The listing builds one solid part. Answer for the finished solid, in the listing's coordinates (mm). Face numbers are marked on the shaded views. A direction names the side the tool comes from. Round coordinates to 2 decimals unless told otherwise and drop trailing zeros. Order: outer loops, then holes, each group sorted by start corner. A loop starts at its lowest first (then second) coordinate and runs counter-clockwise, first axis right, second up. Notation, with made-up numbers: (35.25, 11) -> (49.25, 11) arc R25 cw to (49.25, 50) -> close; hole circle Ø11 at (-27.5, 42.5). An arc over 180 degrees is marked (long way). Return JSON: item names as keys, results as strings. Group by question number.
(1) Each of these flat-tipped pins is pushed along its axis until it touches: pin 1 (9 mm diameter, centred on x = -0.5, y = 68, fed in from +Z); pin 2 (1.5 mm diameter, centred on x = -35.5, z = 3.5, fed in from -Y); pin 3 (11.5 mm diameter, centred on x = 0, y = -70, fed in from -Z); pin 4 (5.5 mm diameter, centred on x = 49.5, y = -49.5, fed in from -Z). Where does it stop, or does it pass through?
(2) Which of the six approach directions +Z, -Z, +X, -X, +Y, -Y give full straight-line access (tool end or side, diameter ignored) to the marked faces 1 and 2?
(3) The part is cut by section D-D (x = -37.5). Determine the outline of the cut face in (y, z), plus the area to 3 significant figures.
(4) The part is cut by section C-C (y = 70). Determine the outline of the cut face in (x, z) (3 decimals).
(5) Consider line 1 (Y direction, x = 0, z = 8.2); line 2 (Y direction, x = -4, z = 7); line 3 (Z direction, x = 38, y = -21). Determine where each line is inside the solid, lowest interval first. Write a range as [from, to].
(6) The part is cut by section A-A (x = 0). Determine the outline of the cut face in (y, z) (3 decimals), plus the area to 3 significant figures.
from build123d import *

# Parameters (mm, degrees)
SKETCH1_R                               = 100
SKETCH1_R_2                             = 40
BOSS_EXTRUDE1_DEPTH                     = 15
CBORE_FOR_M8_HEX_HEAD_BOLT1_D           = 9
CBORE_FOR_M8_HEX_HEAD_BOLT1_CBORE_D     = 18.01
CBORE_FOR_M8_HEX_HEAD_BOLT1_CBORE_DEPTH = 5.68
CIRPATTERN1_COUNT                       = 8
SKETCH5_R                               = 82.5
CUT_EXTRUDE2_DEPTH                      = 5


with BuildPart() as part:
    # Sketch1 → Boss-Extrude1 (new body)
    with BuildSketch(Plane.XY):
        Circle(SKETCH1_R)
        Circle(SKETCH1_R_2, mode=Mode.SUBTRACT)
    extrude(amount=BOSS_EXTRUDE1_DEPTH)

    # CBORE for M8 Hex Head Bolt1 (through all)
    with Locations(Plane.XY.offset(15)):
        with Locations((0, 70)):
            cbore_for_m8_hex_head_bolt1 = CounterBoreHole(CBORE_FOR_M8_HEX_HEAD_BOLT1_D / 2, CBORE_FOR_M8_HEX_HEAD_BOLT1_CBORE_D / 2, CBORE_FOR_M8_HEX_HEAD_BOLT1_CBORE_DEPTH)

    # CirPattern1: CBORE for M8 Hex Head Bolt1 ×8 about axis
    cirpattern1_axis = Axis((0, 0, 0), (0, 0, 1))
    for i in range(1, CIRPATTERN1_COUNT):
        add(cbore_for_m8_hex_head_bolt1.rotate(cirpattern1_axis, i * 360 / CIRPATTERN1_COUNT), mode=Mode.SUBTRACT)

    # Sketch5 → Cut-Extrude2 (cut)
    with BuildSketch(Plane(origin=(0, 0, 0), x_dir=(-1, 0, 0), z_dir=(0, 0, -1))):
        Circle(SKETCH5_R)
    extrude(amount=-CUT_EXTRUDE2_DEPTH, mode=Mode.SUBTRACT)


solid = part.part
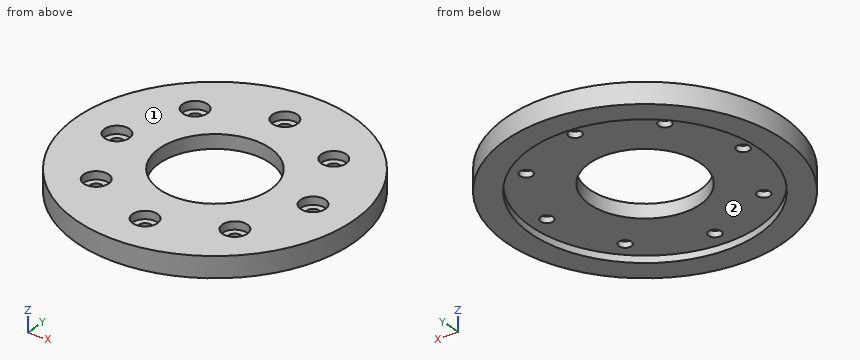
Answer below:
{
 "1": {"pin 1": "stops at z = 9.32", "pin 2": "stops at y = -93.77", "pin 3": "stops at z = 5", "pin 4": "passes through"},
 "2": {"face 1": "+Z, +X, -X, +Y, -Y", "face 2": "-Z"},
 "3": {"outline": "(-92.7, 0) -> (-73.48, 0) -> (-73.48, 5) -> (-13.92, 5) -> (-13.92, 15) -> (-92.7, 15) -> close; (13.92, 5) -> (73.48, 5) -> (73.48, 0) -> (92.7, 0) -> (92.7, 15) -> (13.92, 15) -> close", "area": "1,770 mm²"},
 "4": {"outline": "(-71.414, 0) -> (-43.661, 0) -> (-43.661, 5) -> (-4.5, 5) -> (-4.5, 9.32) -> (-9.005, 9.32) -> (-9.005, 15) -> (-71.414, 15) -> close; (4.5, 5) -> (43.661, 5) -> (43.661, 0) -> (71.414, 0) -> (71.414, 15) -> (9.005, 15) -> (9.005, 9.32) -> (4.5, 9.32) -> close"},
 "5": {"line 1": "y = [-100, -74.5], [-65.5, -40], [40, 65.5], [74.5, 100]", "line 2": "y = [-99.92, -72.06], [-67.94, -39.8], [39.8, 67.94], [72.06, 99.92]", "line 3": "z = [5, 15]"},
 "6": {"outline": "(-100, 0) -> (-82.5, 0) -> (-82.5, 5) -> (-74.5, 5) -> (-74.5, 9.32) -> (-79.005, 9.32) -> (-79.005, 15) -> (-100, 15) -> close; (-65.5, 5) -> (-40, 5) -> (-40, 15) -> (-60.995, 15) -> (-60.995, 9.32) -> (-65.5, 9.32) -> close; (40, 5) -> (65.5, 5) -> (65.5, 9.32) -> (60.995, 9.32) -> (60.995, 15) -> (40, 15) -> close; (74.5, 5) -> (82.5, 5) -> (82.5, 0) -> (100, 0) -> (100, 15) -> (79.005, 15) -> (79.005, 9.32) -> (74.5, 9.32) -> close", "area": "1,090 mm²"}
}
